from build123d import *

# Parameters (mm, degrees)
F0_R          = 131
F0_R_2        = 127
F1_DEPTH      = 4.5
F2_R          = 131
F2_R_2        = 126
F3_DEPTH      = 228.6
F4_R          = 135
F4_R_2        = 126
F5_DEPTH      = 20
F6_R          = 12.5
F7_DEPTH      = 40
F8_R          = 12.5
F9_DEPTH      = 40
F9_DEPTH_BACK = 40


with BuildPart() as f1:
    # F0 (on Top) → F1 (new body)
    with BuildSketch(Plane.XY):
        Circle(F0_R)
        Circle(F0_R_2, mode=Mode.SUBTRACT)
        Circle(F0_R_2)
    extrude(amount=-F1_DEPTH)

    # F2 (on face) → F3 (join)
    with BuildSketch(Plane.XY):
        Circle(F2_R)
        Circle(F2_R_2, mode=Mode.SUBTRACT)
    extrude(amount=F3_DEPTH)

    # F4 (on face) → F5 (join)
    with BuildSketch(Plane.XY.offset(228.6)):
        Circle(F4_R)
        Circle(F4_R_2)
    extrude(amount=F5_DEPTH)

    # F6 (on face) → F7 (join)
    with BuildSketch(Plane.XY.offset(248.6)):
        Circle(F6_R)
    extrude(amount=F7_DEPTH)

    # F8 (on Front) → F9 (join, two sides)
    with BuildSketch(Plane.XZ) as f9_sk:
        with Locations((0, 288.6)):
            Circle(F8_R)
    extrude(amount=-F9_DEPTH)
    extrude(f9_sk.sketch, amount=F9_DEPTH_BACK)


solid = f1.part
Check sheet for the modelled part. Datum: model origin and axes. Units: mm. A direction names the side the tool comes from. Round coordinates to 2 decimals unless told otherwise and drop trailing zeros. Loops run counter-clockwise (first coordinate to the right, second up) from the corner with the lowest first, then second, coordinate; pieces in that order, holes last.
1. Sectioned sample at D-D on z = 177. Record the boundary of the cut face in (x, y), and give its area (3 significant figures).
2. Sectioned sample at A-A on y = 27. Record the boundary of the cut face in (x, z).
3. Mould release check, pull along Z, two halves, no side actions. Record for faces 1 (the flat face through (-2, 2, -4.5)), 2 (the cylindrical face through (-1.627, 0.56, 300.994)), 3 (the flat face through (0, 40, 289)): released by +Z, released by -Z, zero draft, split by the parting line, or undercut.
4. Gauge pin test, flat ends, axial feed: pin 1 Ø7.5 at (x, z) = (0, 290.5) entering from +Y; pin 2 Ø12 at (y, z) = (-30, 222) entering from +X; pin 3 Ø3 at (x, z) = (-7, 248.5) entering from +Y; pin 4 Ø1 at (y, z) = (-66.5, 251) entering from +X. Record the tip position at first contact, or that the pin passes through.
5. Set-up check for faces 4 (the flat face through (0, -40, 289)), 5 (the cylindrical face through (-107.13, -82.15, 238.46)), 6 (the flat face through (-111, 71, 228.6)), 7 (the flat face through (-2, 2, 228.6)): record each of +Z, -Z, +X, -X, +Y, -Y from which the full face is reachable in a straight line by a thin tool's end or side.
6. Sectioned sample at B-B on x = 0. Record the boundary of the cut face in (y, z), and give its area (3 significant figures).
7. Scan lines: probe 1 along Z at (x, y) = (57.5, -94.5); probe 2 along Y at (x, z) = (0, 90); probe 3 along Y at (x, z) = (38, 25). Record each from-to range of solid material in increasing order.
8. Sectioned sample at C-C on y = 0. Record the boundary of the cut face in (x, z), and give its area (3 significant figures).
Recorded:
1. outline: circle Ø262 at (0, 0); hole circle Ø252 at (0, 0)
1. area: 4,040 mm2
2. outline: (-132.27, 228.6) - (-128.19, 228.6) - (-128.19, -4.5) - (128.19, -4.5) - (128.19, 228.6) - (132.27, 228.6) - (132.27, 248.6) - (-132.27, 248.6) - close; circle Ø25 at (0, 288.6); hole (-123.07, 0) - (123.07, 0) - (123.07, 228.6) - (-123.07, 228.6) - close
3. face 1: released by -Z
3. face 2: undercut
3. face 3: zero draft
4. pin 1: stops at y = 40
4. pin 2: stops at x = 128.78
4. pin 3: stops at y = 134.89
4. pin 4: passes through
5. face 4: +Z, +X, -X, -Y
5. face 5: +Z, -Z
5. face 6: -Z
5. face 7: none
6. outline: (-135, 228.6) - (-131, 228.6) - (-131, -4.5) - (131, -4.5) - (131, 228.6) - (135, 228.6) - (135, 248.6) - (12.5, 248.6) - (12.5, 276.1) - (40, 276.1) - (40, 301.1) - (-40, 301.1) - (-40, 276.1) - (-12.5, 276.1) - (-12.5, 248.6) - (-135, 248.6) - close; hole (-126, 0) - (126, 0) - (126, 228.6) - (-126, 228.6) - close
6. area: 11,600 mm2
7. probe 1: z = -4.5 to 0, 228.6 to 248.6
7. probe 2: y = -131 to -126, 126 to 131
7. probe 3: y = -125.37 to -120.13, 120.13 to 125.37
8. outline: (-135, 228.6) - (-131, 228.6) - (-131, -4.5) - (131, -4.5) - (131, 228.6) - (135, 228.6) - (135, 248.6) - (12.5, 248.6) - (12.5, 288.6) arc R12.5 ccw to (-12.5, 288.6) - (-12.5, 248.6) - (-135, 248.6) - close; hole (-126, 0) - (126, 0) - (126, 228.6) - (-126, 228.6) - close
8. area: 10,100 mm2
